Verification items for the finished model (mm, model axes). Face numbers are marked on the shaded views. A direction names the side the tool comes from. Give positions to 0.01 mm unless a question says otherwise; leave off trailing zeros. Order: outer loops, then holes, each group sorted by start corner. A loop starts at its lowest first (then second) coordinate and runs counter-clockwise, first axis right, second up. Notation, with made-up numbers: (87.25, 20) - (140.25, 20) arc R27 ccw to (140.25, 42) - close; hole circle Ø1 at (36.25, 67). An arc over 180 degrees is marked (long way). Answer as a JSON object with one key per item and string values. Group by question number.
(1) Thickness scan on line 1 (X direction, y = 150, z = 30); line 2 (Y direction, x = 15.5, z = -1.5). Record the ranges inside material, lowest first.
(2) Section check A-A (z = 24). Record the boundary of the cut face in (x, y).
(3) Depth check by flat-ended pin: pin 1 Ø22.5 at (y, z) = (137.5, 19.5) entering from +X; pin 2 Ø3 at (y, z) = (22.5, 33.5) entering from -X; pin 3 Ø6 at (x, y) = (1.5, 141.5) entering from -Z. Enter the tip coordinate at first touch or a pass-through.
(4) Access from +Z, -Z, +X, -X, +Y, -Y to the whole of each face (thin tool, end or side, straight path). Record for the marked faces 1, 2, 3 and 4.
(5) Section check B-B (x = 21). Record the boundary of the cut face in (y, z).
(6) Section check D-D (z = -2). Record the boundary of the cut face in (x, y).
(7) Section check C-C (y = 111). Record the boundary of the cut face in (x, z), then the cut area to 4 significant figures.
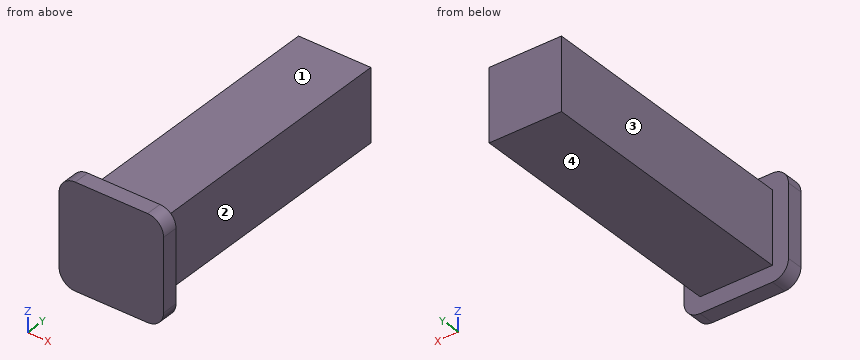
```python
from build123d import *

# Parameters (mm, degrees)
SKETCH1_W           = 45
SKETCH1_H           = 180
BOSS_EXTRUDE1_DEPTH = 45
SKETCH2_W           = 65
SKETCH2_H           = 65
BOSS_EXTRUDE2_DEPTH = 10
FILLET1_R           = 10


with BuildPart() as part:
    # Sketch1 → Boss-Extrude1 (new body)
    with BuildSketch(Plane.XY):
        with Locations((22.5, 90)):
            Rectangle(SKETCH1_W, SKETCH1_H)
    extrude(amount=BOSS_EXTRUDE1_DEPTH)

    # Sketch2 → Boss-Extrude2 (add)
    with BuildSketch(Plane.XZ):
        with Locations((22.5, 22.5)):
            Rectangle(SKETCH2_W, SKETCH2_H)
    extrude(amount=-BOSS_EXTRUDE2_DEPTH)

    # Fillet1
    fillet1_edges = [part.edges().sort_by_distance(p)[0] for p in [
        (-10, 5, -10),
        (-10, 5, 55),
        (55, 5, 55),
        (55, 5, -10),
    ]]
    fillet(fillet1_edges, radius=FILLET1_R)


solid = part.part
```
Solutions:
{
 "1": {"line 1": "x = 0 to 45", "line 2": "y = 0 to 10"},
 "2": {"outline": "(-10, 0) - (55, 0) - (55, 10) - (45, 10) - (45, 180) - (0, 180) - (0, 10) - (-10, 10) - close"},
 "3": {"pin 1": "stops at x = 45", "pin 2": "stops at x = 0", "pin 3": "stops at z = 0"},
 "4": {"face 1": "+Z, +X, -X, +Y", "face 2": "+Z, -Z, +X, +Y", "face 3": "+Z, -Z, -X, +Y", "face 4": "-Z, +X, -X, +Y"},
 "5": {"outline": "(0, -10) - (10, -10) - (10, 0) - (180, 0) - (180, 45) - (10, 45) - (10, 55) - (0, 55) - close"},
 "6": {"outline": "(-9.8, 0) - (54.8, 0) - (54.8, 10) - (-9.8, 10) - close"},
 "7": {"outline": "(0, 0) - (45, 0) - (45, 45) - (0, 45) - close", "area": "2,025 mm2"}
}
